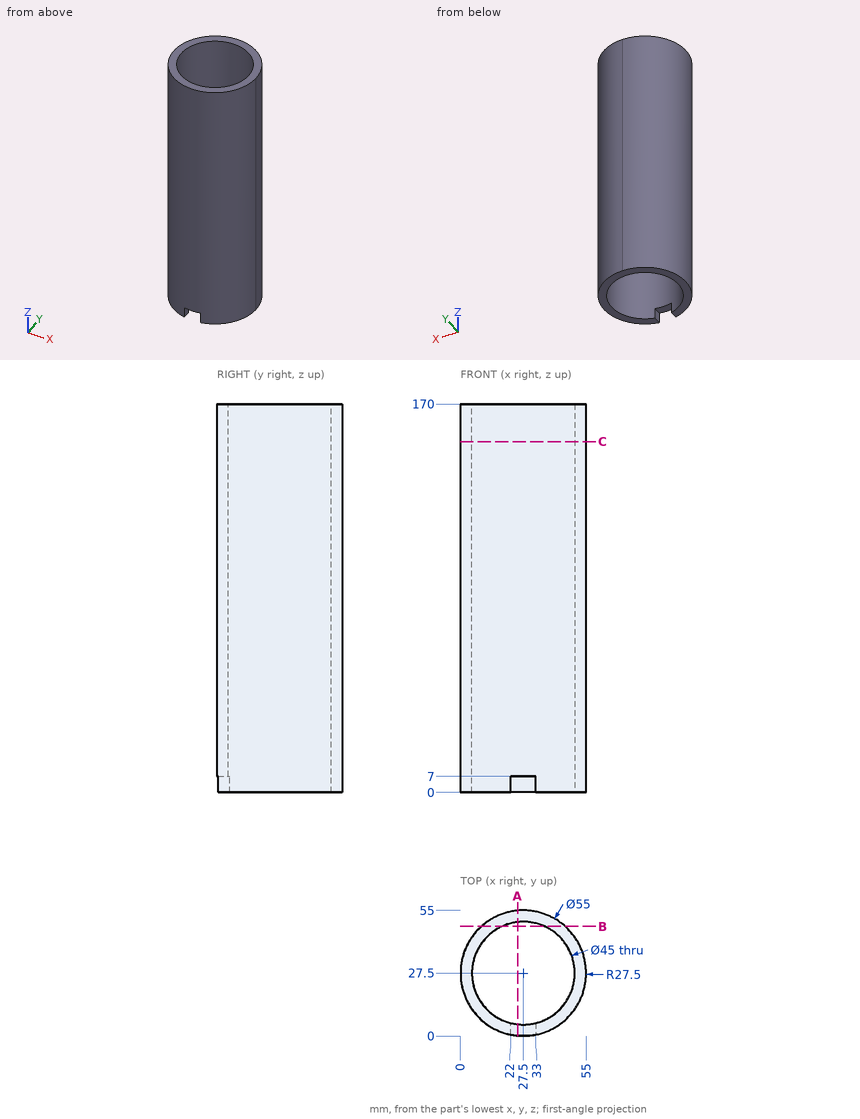
Input: dimensioned drawing with shaded views. Units: mm. Origin: part minimum x, y, z. Round coordinates to 2 decimals unless told otherwise and drop trailing zeros. Order: outer loops, then holes, each group sorted by start corner. A loop starts at its lowest first (then second) coordinate and runs counter-clockwise, first axis right, second up. Notation, with made-up numbers: (19, 16) -> (34, 16) arc R36 cw to (34, 52) -> close; hole circle Ø2 at (-28.5, 17.5). An arc over 180 degrees is marked (long way). One line per item, written item: value. Start each with the question number.
Q1. Pin query (flat end, axial travel): pin 1 (12 mm diameter, centred on x = 16.5, z = 84.5, fed in from -Y); pin 2 (1.7 mm diameter, centred on x = 26.5, y = 3, fed in from -Z); pin 3 (4 mm diameter, centred on y = 39.5, z = 66, fed in from -X). Return the tip coordinate at first contact, or that it passes through.
Q2. Section query A-A (x = 25). Return the cut outline in (y, z), plus the area to 3 significant figures.
Q3. Material intervals for probe 1 along Y at (x, z) = (27, 118); probe 2 along Y at (x, z) = (44, 128), sorted ascending.
Q4. Section query C-C (z = 153.5). Return the cut outline in (x, y).
Q5. Section query B-B (y = 48). Return the cut outline in (x, z).
Findings below:
1. pin 1: y = 0.46
1. pin 2: z = 7
1. pin 3: x = 1.88
2. outline: (0.11, 7) -> (5.14, 7) -> (5.14, 170) -> (0.11, 170) -> close; (49.86, 0) -> (54.89, 0) -> (54.89, 170) -> (49.86, 170) -> close
2. area: 1,670 mm²
3. probe 1: 0 to 5.01, 49.99 to 55
3. probe 2: 5.5 to 12.2, 42.8 to 49.5
4. outline: circle Ø55 at (27.5, 27.5); hole circle Ø45 at (27.5, 27.5)
5. outline: (9.17, 0) -> (18.23, 0) -> (18.23, 170) -> (9.17, 170) -> close; (36.77, 0) -> (45.83, 0) -> (45.83, 170) -> (36.77, 170) -> close
